Read the model definition and answer for the solid it produces. Units are mm, in the model's axes. Face numbers are marked on the shaded views. Round coordinates to 2 decimals unless told otherwise and drop trailing zeros. Order: outer loops, then holes, each group sorted by start corner. A loop starts at its lowest first (then second) coordinate and runs counter-clockwise, first axis right, second up. Notation, with made-up numbers: M 88.25,78.25 L 119.25,78.25 A12 cw 119.25,83.25 Z; hole C 42.25,80.25 d5. An arc over 180 degrees is marked long. Answer as CSV lines item,"result".
```python
from build123d import *

# Parameters (mm, degrees)
CHAMFER1_SIZE = 0.15
FILLET1_R     = 0.15


with BuildPart() as part:
    # Sketch3 → Revolve1 (revolve)
    with BuildSketch(Plane(origin=(0, 0, 0), x_dir=(0, 0, -1), z_dir=(1, 0, 0))):
        Polygon((3, 6), (1, 6), (1, 5.0255), (-3, 5.0255), (-3, 3), (3, 3), align=None)
    revolve(axis=Axis((0, 0, -3), (0, 0, 1)))

    # Chamfer1
    chamfer1_edges = [part.edges().sort_by_distance(p)[0] for p in [
        (0, -3, 3),
        (0, -5.0255, 3),
        (0, -6, -1),
        (0, -6, -3),
    ]]
    chamfer(chamfer1_edges, length=CHAMFER1_SIZE)

    # Fillet1
    fillet1_edges = [part.edges().sort_by_distance(p)[0] for p in [
        (0, -5.0255, -1),
    ]]
    fillet(fillet1_edges, radius=FILLET1_R)


solid = part.part
```
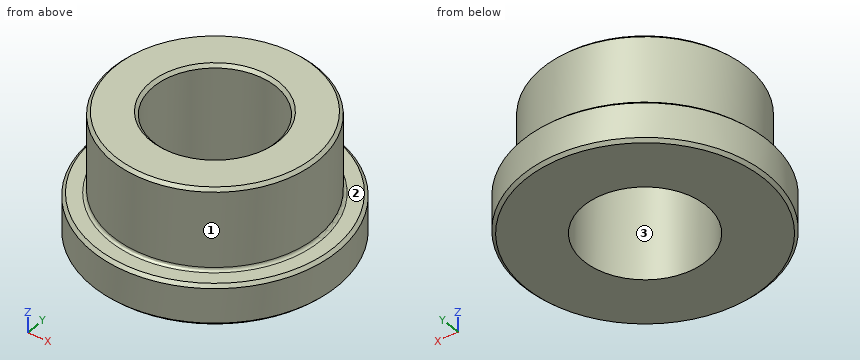
Item 1: Flat-ended cylindrical pins translate along their axes: pin 1 (1.5 mm diameter, centred on y = 2, z = -1.5, fed in from -X); pin 2 (1.5 mm diameter, centred on y = 4.5, z = 0, fed in from -X). Find the tip coordinate at first contact, or state that the pin passes through.
Ans:
pin 1,"x = -5.87"
pin 2,"x = -3.35"
Item 2: A cutting plane is placed at A-A, the plane y = 0. Determine the outline of the cut face in (x, z).
Ans:
outline,"M -6,-2.85 L -5.85,-3 L -3,-3 L -3,2.85 L -3.15,3 L -4.88,3 L -5.03,2.85 L -5.03,-0.85 A0.15 cw -5.18,-1 L -5.85,-1 L -6,-1.15 Z; M 3,-3 L 5.85,-3 L 6,-2.85 L 6,-1.15 L 5.85,-1 L 5.18,-1 A0.15 cw 5.03,-0.85 L 5.03,2.85 L 4.88,3 L 3.15,3 L 3,2.85 Z"
Item 3: Find the intervals of material crossed by probe 1 along X at (y, z) = (0, 0.6); probe 2 along X at (y, z) = (0, -1.55), in increasing order. Write a range as [from, to].
Ans:
probe 1,"[-5.03, -3], [3, 5.03]"
probe 2,"[-6, -3], [3, 6]"
Item 4: A cutting plane is placed at C-C, the plane z = -0.2. Determine the outline of the cut face in (x, y).
Ans:
outline,"C 0,0 d10.05; hole C 0,0 d6"
Item 5: Determine the mould class of the marked faces 1, 2 and 3 for opening direction Y: +Y half, -Y half, draft (parallel to the pull), parting line (faces both ways), or undercut.
Ans:
face 1,"parting line"
face 2,"draft"
face 3,"undercut"
